Source: three-view drawing plus pictorial views. Frame: mm from the lowest corner of the part. A direction names the side the tool comes from. Round coordinates to 2 decimals unless told otherwise and drop trailing zeros. Order: outer loops, then holes, each group sorted by start corner. A loop starts at its lowest first (then second) coordinate and runs counter-clockwise, first axis right, second up. Notation, with made-up numbers: M 42,68 L 94,68 A19 ccw 94,82 Z; hole C -29,18.5 d11. An arc over 180 degrees is marked long. Return JSON: item names as keys, results as strings. Group by question number.
Q1. Ray query, probe 1 along Z at (x, y) = (12, 80); probe 2 along Y at (x, z) = (3.5, 55.5); probe 3 along Z at (x, y) = (45, 39.5). Return the intervals inside material, ascending.
Q2. Contact query for flat-ended pins moving along their axis: pin 1 (10 mm diameter, centred on y = 43, z = 38.5, fed in from -X); pin 2 (5 mm diameter, centred on x = 19.5, y = 3, fed in from +Z); pin 3 (6 mm diameter, centred on x = 24, z = 36, fed in from -Y). Output: stop coordinate, or through.
Q3. Access query for the marked faces 1, 2, 3, 4 and 5. Directions: +Z, -Z, +X, -X, +Y, -Y. A direction counts if a zero-diameter tool reaches every point of the face in a straight line with its end or side. Return the directions, or none.
Q4. Mould query, pull axis Y, two halves, no side actions, for the marked faces 6, 7 and 8. Classes: released by +Y, released by -Y, zero draft, split by the parting line, or undercut.
Q5. Cut plane A-A on x = 25. Output: boundary loops of the cut face in (y, z), and give its area (4 significant figures).
Q6. Cut plane C-C on y = 71. Output: boundary loops of the cut face in (x, z), and give its area (3 significant figures).
Q7. Cut plane D-D on x = 5. Output: boundary loops of the cut face in (y, z).
Q8. Cut plane B-B on z = 38. Output: boundary loops of the cut face in (x, y), and give its area (3 significant figures).
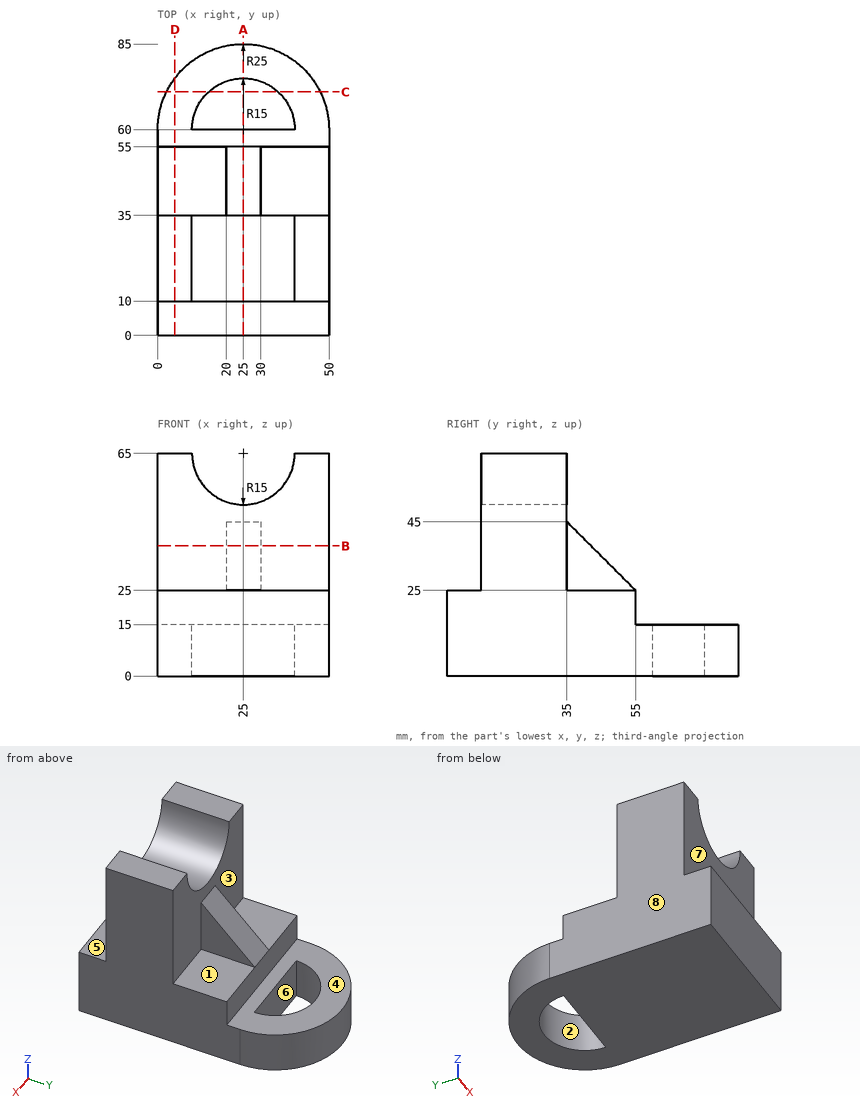
Result sheet:
{
 "1": {"probe 1": "z = 0 to 15", "probe 2": "y = 10 to 35", "probe 3": "z = 0 to 25"},
 "2": {"pin 1": "stops at x = 20", "pin 2": "stops at z = 25", "pin 3": "stops at y = 10"},
 "3": {"face 1": "+Z, +X, +Y", "face 2": "+Z, -Z", "face 3": "+Z, +Y", "face 4": "+Z, +X, -X, +Y", "face 5": "+Z, +X, -X, -Y"},
 "4": {"face 6": "undercut", "face 7": "released by -Y", "face 8": "zero draft"},
 "5": {"outline": "M 0,0 L 60,0 L 60,15 L 55,15 L 55,25 L 35,45 L 35,50 L 10,50 L 10,25 L 0,25 Z; M 75,0 L 85,0 L 85,15 L 75,15 Z", "area": "2,425 mm²"},
 "6": {"outline": "M 2.55,0 L 14.8,0 L 14.8,15 L 2.55,15 Z; M 35.2,0 L 47.45,0 L 47.45,15 L 35.2,15 Z", "area": "368 mm²"},
 "7": {"outline": "M 0,0 L 75,0 L 75,15 L 55,15 L 55,25 L 35,25 L 35,65 L 10,65 L 10,25 L 0,25 Z"},
 "8": {"outline": "M 0,10 L 50,10 L 50,35 L 30,35 L 30,42 L 20,42 L 20,35 L 0,35 Z", "area": "1,320 mm²"}
}
